Autodesk Inventor part; units mm, degrees
ref_plane "to_parts_XY" through (0, 0, -200) normal (0, 0, 1) x (1, 0, 0)
ref_plane "to_parts_YZ" through (0, 0, -200) normal (1, 0, 0) x (0, 1, 0)
ref_plane "to_parts_ZX" through (0, 0, -200) normal (0, 1, 0) x (0, 0, 1)
sketch "Sketch_1" plane through (0, 0, 0) normal (0, 0, 1) x (1, 0, 0)
  line L0 (-20, 16.83) -> (-20, 5.6904)
  arc A0 (-20, 5.6904) -> (-18.43, 4.1204) centre (-18.43, 5.6904) ccw
  line L1 (-18.43, 4.1204) -> (-17.25, 4.1204)
  arc A1 (-17.25, 4.1204) -> (-15.68, 5.6904) centre (-17.25, 5.6904) ccw
  line L2 (-15.68, 5.6904) -> (-15.68, 8.7154)
  arc A2 (-14.11, 10.2854) -> (-15.68, 8.7154) centre (-14.11, 8.7154) ccw
  line L3 (-14.11, 10.2854) -> (-13.6549, 10.2854)
  arc A3 (-13.1175, 10.0628) -> (-13.6549, 10.2854) centre (-13.6549, 9.5254) ccw
  line L4 (-13.1175, 10.0628) -> (-9.1098, 6.0551)
  arc A4 (-7.685, 2.6153) -> (-9.1098, 6.0551) centre (-12.5496, 2.6153) ccw
  line L5 (-7.685, 2.6153) -> (-7.685, -2.6153)
  arc A5 (-9.1098, -6.0551) -> (-7.685, -2.6153) centre (-12.5496, -2.6153) ccw
  line L6 (-9.1098, -6.0551) -> (-13.1175, -10.0628)
  arc A6 (-13.6549, -10.2854) -> (-13.1175, -10.0628) centre (-13.6549, -9.5254) ccw
  line L7 (-13.6549, -10.2854) -> (-14.11, -10.2854)
  arc A7 (-15.68, -8.7154) -> (-14.11, -10.2854) centre (-14.11, -8.7154) ccw
  line L8 (-15.68, -8.7154) -> (-15.68, -5.6904)
  arc A8 (-15.68, -5.6904) -> (-17.25, -4.1204) centre (-17.25, -5.6904) ccw
  line L9 (-17.25, -4.1204) -> (-18.43, -4.1204)
  arc A9 (-18.43, -4.1204) -> (-20, -5.6904) centre (-18.43, -5.6904) ccw
  line L10 (-20, -5.6904) -> (-20, -16.83)
  arc A10 (-20, -16.83) -> (-16.83, -20) centre (-16.83, -16.83) ccw
  line L11 (-16.83, -20) -> (-5.6904, -20)
  arc A11 (-5.6904, -20) -> (-4.1204, -18.43) centre (-5.6904, -18.43) ccw
  line L12 (-4.1204, -18.43) -> (-4.1204, -17.25)
  arc A12 (-4.1204, -17.25) -> (-5.6904, -15.68) centre (-5.6904, -17.25) ccw
  line L13 (-5.6904, -15.68) -> (-8.7154, -15.68)
  arc A13 (-10.2854, -14.11) -> (-8.7154, -15.68) centre (-8.7154, -14.11) ccw
  line L14 (-10.2854, -14.11) -> (-10.2854, -13.6549)
  arc A14 (-10.0628, -13.1175) -> (-10.2854, -13.6549) centre (-9.5254, -13.6549) ccw
  line L15 (-10.0628, -13.1175) -> (-6.0551, -9.1098)
  arc A15 (-2.6153, -7.685) -> (-6.0551, -9.1098) centre (-2.6153, -12.5496) ccw
  line L16 (-2.6153, -7.685) -> (2.6153, -7.685)
  arc A16 (6.0551, -9.1098) -> (2.6153, -7.685) centre (2.6153, -12.5496) ccw
  line L17 (6.0551, -9.1098) -> (10.0628, -13.1175)
  arc A17 (10.2854, -13.6549) -> (10.0628, -13.1175) centre (9.5254, -13.6549) ccw
  line L18 (10.2854, -13.6549) -> (10.2854, -14.11)
  arc A18 (8.7154, -15.68) -> (10.2854, -14.11) centre (8.7154, -14.11) ccw
  line L19 (8.7154, -15.68) -> (5.6904, -15.68)
  arc A19 (5.6904, -15.68) -> (4.1204, -17.25) centre (5.6904, -17.25) ccw
  line L20 (4.1204, -17.25) -> (4.1204, -18.43)
  arc A20 (4.1204, -18.43) -> (5.6904, -20) centre (5.6904, -18.43) ccw
  line L21 (5.6904, -20) -> (16.83, -20)
  arc A21 (16.83, -20) -> (20, -16.83) centre (16.83, -16.83) ccw
  line L22 (20, -16.83) -> (20, -5.6904)
  arc A22 (20, -5.6904) -> (18.43, -4.1204) centre (18.43, -5.6904) ccw
  line L23 (18.43, -4.1204) -> (17.25, -4.1204)
  arc A23 (17.25, -4.1204) -> (15.68, -5.6904) centre (17.25, -5.6904) ccw
  line L24 (15.68, -5.6904) -> (15.68, -8.7154)
  arc A24 (14.11, -10.2854) -> (15.68, -8.7154) centre (14.11, -8.7154) ccw
  line L25 (14.11, -10.2854) -> (13.6549, -10.2854)
  arc A25 (13.1175, -10.0628) -> (13.6549, -10.2854) centre (13.6549, -9.5254) ccw
  line L26 (13.1175, -10.0628) -> (9.1098, -6.0551)
  arc A26 (7.685, -2.6153) -> (9.1098, -6.0551) centre (12.5496, -2.6153) ccw
  line L27 (7.685, -2.6153) -> (7.685, 2.6153)
  arc A27 (9.1098, 6.0551) -> (7.685, 2.6153) centre (12.5496, 2.6153) ccw
  line L28 (9.1098, 6.0551) -> (13.1175, 10.0628)
  arc A28 (13.6549, 10.2854) -> (13.1175, 10.0628) centre (13.6549, 9.5254) ccw
  line L29 (13.6549, 10.2854) -> (14.11, 10.2854)
  arc A29 (15.68, 8.7154) -> (14.11, 10.2854) centre (14.11, 8.7154) ccw
  line L30 (15.68, 8.7154) -> (15.68, 5.6904)
  arc A30 (15.68, 5.6904) -> (17.25, 4.1204) centre (17.25, 5.6904) ccw
  line L31 (17.25, 4.1204) -> (18.43, 4.1204)
  arc A31 (18.43, 4.1204) -> (20, 5.6904) centre (18.43, 5.6904) ccw
  line L32 (20, 5.6904) -> (20, 16.83)
  arc A32 (20, 16.83) -> (16.83, 20) centre (16.83, 16.83) ccw
  line L33 (16.83, 20) -> (5.6904, 20)
  arc A33 (5.6904, 20) -> (4.1204, 18.43) centre (5.6904, 18.43) ccw
  line L34 (4.1204, 18.43) -> (4.1204, 17.25)
  arc A34 (4.1204, 17.25) -> (5.6904, 15.68) centre (5.6904, 17.25) ccw
  line L35 (5.6904, 15.68) -> (8.7154, 15.68)
  arc A35 (10.2854, 14.11) -> (8.7154, 15.68) centre (8.7154, 14.11) ccw
  line L36 (10.2854, 14.11) -> (10.2854, 13.6549)
  arc A36 (10.0628, 13.1175) -> (10.2854, 13.6549) centre (9.5254, 13.6549) ccw
  line L37 (10.0628, 13.1175) -> (6.0551, 9.1098)
  arc A37 (2.6153, 7.685) -> (6.0551, 9.1098) centre (2.6153, 12.5496) ccw
  line L38 (2.6153, 7.685) -> (-2.6153, 7.685)
  arc A38 (-6.0551, 9.1098) -> (-2.6153, 7.685) centre (-2.6153, 12.5496) ccw
  line L39 (-6.0551, 9.1098) -> (-10.0628, 13.1175)
  arc A39 (-10.2854, 13.6549) -> (-10.0628, 13.1175) centre (-9.5254, 13.6549) ccw
  line L40 (-10.2854, 13.6549) -> (-10.2854, 14.11)
  arc A40 (-8.7154, 15.68) -> (-10.2854, 14.11) centre (-8.7154, 14.11) ccw
  line L41 (-8.7154, 15.68) -> (-5.6904, 15.68)
  arc A41 (-5.6904, 15.68) -> (-4.1204, 17.25) centre (-5.6904, 17.25) ccw
  line L42 (-4.1204, 17.25) -> (-4.1204, 18.43)
  arc A42 (-4.1204, 18.43) -> (-5.6904, 20) centre (-5.6904, 18.43) ccw
  line L43 (-5.6904, 20) -> (-16.83, 20)
  arc A43 (-16.83, 20) -> (-20, 16.83) centre (-16.83, 16.83) ccw
  circle A44 centre (0, 0) radius 3.4
extrude "Extrusion1" add sketch "Sketch_1" against normal blind 400
ref_plane "to_parts_XY" through (0, 0, -200) normal (0, 0, 1) x (1, 0, 0)
ref_plane "to_parts_YZ" through (0, 0, -200) normal (1, 0, 0) x (0, 1, 0)
ref_plane "to_parts_ZX" through (0, 0, -200) normal (0, 1, 0) x (0, 0, 1)
properties part number "40-4040-400-CL"
For this review, take the finished solid that the model builds, in its own axes (mm). Give positions to 0.01 mm unless a question says otherwise; leave off trailing zeros. Answer as a JSON object with one key per item and string values. Group by question number.
Item 1: Clearance check with flat-ended pins moving along their axes: pin 1 Ø1 at (x, z) = (-2.5, -325) entering from +Y; pin 2 Ø4 at (x, z) = (-1, -220.5) entering from -Y; pin 3 Ø5 at (x, y) = (7.5, -11) entering from -Z; pin 4 Ø0.9 at (y, z) = (-18, -171.5) entering from -X. State where each tip first meets the part, or that it passes through.
Item 2: Wall thickness on line 1 along Y through (x, z) = (7, -250); line 2 along Y through (x, z) = (0, -93) (3 decimals); line 3 along Y through (x, z) = (-6.5, -324.5): over which ranges is each line inside the solid? List them lowest first.
Item 3: Draft analysis for pull direction X (two halves, no side actions). For faces 1 (the cylindrical face through (-0.74, -3.32, -197.2)), 2 (the flat face through (4, 0, 0)), 3 (the flat face through (-20, 11, -197)), 4 (the flat face through (20, -11, -197)), state which applies: pulls with the +X half, pulls with the -X half, needs draft (parallel to the pull), parting line crosses it, or undercut.
Reported:
{
 "1": {"pin 1": "y = 7.7", "pin 2": "y = -7.7", "pin 3": "z = -400", "pin 4": "x = -19.92"},
 "2": {"line 1": "-20 to -15.68, -10.05 to 10.05, 15.68 to 20", "line 2": "-7.685 to -3.4, 3.4 to 7.685", "line 3": "-20 to -15.68, -9.55 to 9.55, 15.68 to 20"},
 "3": {"face 1": "undercut", "face 2": "needs draft", "face 3": "pulls with the -X half", "face 4": "pulls with the +X half"}
}
